Work out the finished part from the listing and answer in its coordinate system (mm). A direction names the side the tool comes from. Give positions to 0.01 mm unless a question says otherwise; leave off trailing zeros. Loops run counter-clockwise (first coordinate to the right, second up) from the corner with the lowest first, then second, coordinate; pieces in that order, holes last. Notation, with made-up numbers: M 85,22.5 L 134,22.5 A16 ccw 134,46.5 Z; hole C 61,21 d3. An arc over 180 degrees is marked long. Answer as a JSON object with one key per item and string values. Group by question number.
```python
from build123d import *

# Parameters (mm, degrees)
F1_DEPTH = 5
F2_DEPTH = 5
F3_SIZE2 = 10
F3_SIZE  = 5
F4_D     = 2.5908
F4_DEPTH = 5.001


with BuildPart() as f1:
    # F0 (on Top) → F1 (new body)
    with BuildSketch(Plane.XY):
        with BuildLine():
            ThreePointArc((-74.419728056, -63.7628738065), (-71.7533661722, -66.7491905791), (-68.9672591452, -69.6241133947))
            Line((-68.9672591452, -69.6241133947), (-56.6715728753, -57.3284271247))
            ThreePointArc((-56.6715728753, -57.3284271247), (-56.6715728753, -51.6715728753), (-62.3284271247, -51.6715728753))
            Line((-62.3284271247, -51.6715728753), (-74.419728056, -63.7628738065))
        make_face()
    extrude(amount=F1_DEPTH)

    # F0 (on Top) → F2 (join)
    with BuildSketch(Plane.XY):
        with BuildLine():
            ThreePointArc((-74.419728056, -63.7628738065), (-71.7533661722, -66.7491905791), (-68.9672591452, -69.6241133947))
            Line((-68.9672591452, -69.6241133947), (-56.6715728753, -57.3284271247))
            ThreePointArc((-56.6715728753, -57.3284271247), (-56.6715728753, -51.6715728753), (-62.3284271247, -51.6715728753))
            Line((-62.3284271247, -51.6715728753), (-74.419728056, -63.7628738065))
        make_face()
    extrude(amount=-F2_DEPTH)

    # F3
    f3_edges = [f1.edges().sort_by_distance(p)[0] for p in [
        (-71.753366, -66.749191, -5),
    ]]
    f3_side = f1.faces().sort_by_distance((-71.753366, -66.749191, 0))[0]
    chamfer(f3_edges, length=F3_SIZE, length2=F3_SIZE2, reference=f3_side)

    # F4 (through all, one way)
    with BuildSketch(Plane.XY):
        with Locations((-59.5, -54.5)):
            Circle(F4_D / 2)
    extrude(amount=-F4_DEPTH, mode=Mode.SUBTRACT)


solid = f1.part
```
Item 1: Find the intervals of material crossed by probe 1 along Z at (x, y) = (-58.5, -53.75); probe 2 along Y at (x, z) = (-59.5, -2.4); probe 3 along Z at (x, y) = (-67.25, -63.5), in increasing order. Write a range as [from, to].
Item 2: A cutting plane is placed at A-A (x = -60). Determine the outline of the cut face in (y, z), and give its area (3 significant figures).
Item 3: A tool of negligible diameter and unlimited length cuts with its end or side. For faces 1 (the flat face through (-60, -54, 0)), 2 (the flat face through (-62.905, -63.562, 0.07)), from which of +Z, -Z, +X, -X, +Y, -Y can it reach the whole face along a straight path? Write none if from no direction.
Item 4: A cutting plane is placed at C-C (z = -1.5). Determine the outline of the cut face in (x, y), and give its area (3 significant figures).
Item 5: A cutting plane is placed at B-B (y = -54). Determine the outline of the cut face in (x, z).
Item 6: Given pin 1 Ø3 at (x, z) = (-65.5, 0) entering from +Y; pin 2 Ø1 at (x, z) = (-66, 1) entering from -Y; pin 3 Ø2 at (x, z) = (-64.5, 2) entering from -Y, each flat-ended and moving along its own axis, determine where each tip first touches the part or whether it passes through.
Item 7: A cutting plane is placed at D-D (z = 3.25). Determine the outline of the cut face in (x, y), and give its area (3 significant figures).
The answers:
{
 "1": {"probe 1": "z = [0, 5]", "probe 2": "y = [-60.16, -55.8], [-53.2, -50.5]", "probe 3": "z = [-2.75, 5]"},
 "2": {"outline": "M -60.66,-5 L -55.7,-5 L -55.7,0 L -53.3,0 L -53.3,-5 L -50.53,-5 L -50.53,5 L -60.66,5 Z", "area": "89.3 mm^2"},
 "3": {"face 1": "-Z", "face 2": "+Z, -Z, +X, -Y"},
 "4": {"outline": "M -72.29,-61.64 A95 ccw -66.85,-67.5 L -56.67,-57.33 A4 ccw -62.33,-51.67 Z; hole C -59.5,-54.5 d2.59", "area": "134 mm^2"},
 "5": {"outline": "M -64.66,-5 L -60.7,-5 L -60.7,0 L -58.3,0 L -58.3,-5 L -55.53,-5 L -55.53,5 L -64.66,5 Z"},
 "6": {"pin 1": "stops at y = -53.34", "pin 2": "stops at y = -67.16", "pin 3": "stops at y = -66.16"},
 "7": {"outline": "M -74.42,-63.76 A98 ccw -68.97,-69.62 L -56.67,-57.33 A4 ccw -62.33,-51.67 Z", "area": "164 mm^2"}
}
